Here's how the part is built. I have some questions about the finished solid (model axes, mm). A direction names the side the tool comes from. Give positions to 0.01 mm unless a question says otherwise; leave off trailing zeros. Order: outer loops, then holes, each group sorted by start corner. A loop starts at its lowest first (then second) coordinate and runs counter-clockwise, first axis right, second up.
from build123d import *

# Parameters (mm, degrees)
SKETCH1_W           = 94
SKETCH1_H           = 28
BOSS_EXTRUDE1_DEPTH = 25
FILLET1_R           = 10
SKETCH2_W           = 13
SKETCH2_H           = 9.5
BOSS_EXTRUDE2_DEPTH = 10


with BuildPart() as part:
    # Sketch1 → Boss-Extrude1 (new body)
    with BuildSketch(Plane.XY):
        Rectangle(SKETCH1_W, SKETCH1_H)
    extrude(amount=BOSS_EXTRUDE1_DEPTH)

    # Fillet1
    fillet1_edges = [part.edges().sort_by_distance(p)[0] for p in [
        (-47, 0, 25),
        (47, 0, 25),
    ]]
    fillet(fillet1_edges, radius=FILLET1_R)

    # Sketch2 → Boss-Extrude2 (add)
    with BuildSketch(Plane(origin=(0, 0, 0), x_dir=(-1, 0, 0), z_dir=(0, 0, -1))):
        with Locations((-13.5, -3.75)):
            Rectangle(SKETCH2_W, SKETCH2_H)
    extrude(amount=BOSS_EXTRUDE2_DEPTH)


solid = part.part
Q1. If we section it at C-C on z = 21: List the corners of the cut face in (x, y) for me, plus the area to 3 significant figures.
Filled sheet:
outline: (-45, -14) - (45, -14) - (45, 14) - (-45, 14) - close
area: 2,520 mm2
Q2. If we section it at A-A on x = 16.5: List the corners of the cut face in (y, z) for me.
Filled sheet:
outline: (-14, 0) - (-8.5, 0) - (-8.5, -10) - (1, -10) - (1, 0) - (14, 0) - (14, 25) - (-14, 25) - close
Q3. If we section it at D-D on x = -4.5: List the corners of the cut face in (y, z) for me, plus the area to 3 significant figures.
Filled sheet:
outline: (-14, 0) - (14, 0) - (14, 25) - (-14, 25) - close
area: 700 mm2
Q4. If we section it at B-B on y = -6: List the corners of the cut face in (x, z) for me, plus the area to 3 significant figures.
Filled sheet:
outline: (-47, 0) - (7, 0) - (7, -10) - (20, -10) - (20, 0) - (47, 0) - (47, 15) arc R10 ccw to (37, 25) - (-37, 25) arc R10 ccw to (-47, 15) - close
area: 2,440 mm2
Q5. For faces 1 (the face through (14, 1, -5)), 2 (the face through (-44.15, 0.2, 21.99)), 3 (the face through (14, -8.5, -5)), 4 (the face through (20, -4, -5)), 5 (the face through (7, -4, -5)), which set-ups out of +Z, -Z, +X, -X, +Y, -Y let a thin tool reach every point of the face, with its end or its side?
Filled sheet:
face 1: -Z, +X, -X, +Y
face 2: +Z, -X, +Y, -Y
face 3: -Z, +X, -X, -Y
face 4: -Z, +X, +Y, -Y
face 5: -Z, -X, +Y, -Y
Q6. I need wall thicknesses on L1, parallel to X at y = -8, z = -7; L2, parallel to Z at x = 34, y = -4.5; L3, parallel to X at y = -5.75, z = 19.5. Which ranges of each line are inside material? Lowest first, please.
Filled sheet:
L1: x = 7 to 20
L2: z = 0 to 25
L3: x = -45.93 to 45.93
Q7. I'm going to push flat-ended pins straight in: P1, Ø2, axis at x = -17, y = 9, coming from the -Z side; P2, Ø3, axis at y = -2.5, z = -7.5, coming from the +X side; P3, Ø5, axis at x = 10.5, z = -3, coming from the +Y side. Where does each tip first touch, or does it pass through?
Filled sheet:
P1: stops at z = 0
P2: stops at x = 20
P3: stops at y = 1
